Geometry: final body of the model. Coordinates: model frame, mm. A direction names the side the tool comes from. Round coordinates to 2 decimals unless told otherwise and drop trailing zeros. Loops run counter-clockwise (first coordinate to the right, second up) from the corner with the lowest first, then second, coordinate; pieces in that order, holes last. Notation, with made-up numbers: (36, 60) -> (78, 60) arc R5 cw to (78, 64) -> close; hole circle Ø1 at (19, 50). An arc over 180 degrees is marked (long way). Answer in a Markdown table with one row per item.
```python
from build123d import *

# Parameters (mm, degrees)
SKETCH1_W           = 30.1
SKETCH1_H           = 25.3
BOSS_EXTRUDE1_DEPTH = 1.1
SKETCH2_R           = 1.05
CUT_EXTRUDE1_DEPTH  = 2.1
SKETCH3_W           = 13
SKETCH3_H           = 13
BOSS_EXTRUDE2_DEPTH = 3
BOSS_EXTRUDE3_DEPTH = 3
SKETCH5_R           = 6.85
BOSS_EXTRUDE4_DEPTH = 20


with BuildPart() as part:
    # Sketch1 → Boss-Extrude1 (new body)
    with BuildSketch(Plane.XY):
        Rectangle(SKETCH1_W, SKETCH1_H)
    extrude(amount=BOSS_EXTRUDE1_DEPTH)

    # Sketch2 → Cut-Extrude1 (cut, through all)
    with BuildSketch(Plane.XY.offset(1.1)):
        with Locations((-11.8, 11.9)):
            Circle(SKETCH2_R)
        with Locations((11.8, 11.9)):
            Circle(SKETCH2_R)
        with Locations((11.8, -11.9)):
            Circle(SKETCH2_R)
        with Locations((-11.8, -11.9)):
            Circle(SKETCH2_R)
    extrude(amount=-CUT_EXTRUDE1_DEPTH, mode=Mode.SUBTRACT)

    # Sketch3 → Boss-Extrude2 (add)
    with BuildSketch(Plane.XY.offset(1.1)):
        Rectangle(SKETCH3_W, SKETCH3_H)
    extrude(amount=BOSS_EXTRUDE2_DEPTH)

    # Sketch4 → Boss-Extrude3 (add)
    with BuildSketch(Plane.XY.offset(1.1)):
        with BuildLine():
            Line((-8.9, 2), (8.9, 2))
            ThreePointArc((8.9, 2), (10.9, 0), (8.9, -2))
            Line((8.9, -2), (-8.9, -2))
            ThreePointArc((-8.9, -2), (-10.9, 0), (-8.9, 2))
        make_face()
    extrude(amount=BOSS_EXTRUDE3_DEPTH)

    # Sketch5 → Boss-Extrude4 (add)
    with BuildSketch(Plane.XY.offset(1.1)):
        Circle(SKETCH5_R)
    extrude(amount=BOSS_EXTRUDE4_DEPTH)


solid = part.part
```
Item 1: Pin query (flat end, axial travel): pin 1 Ø12 at (x, z) = (11.5, 12.5) entering from +Y; pin 2 Ø1.2 at (x, y) = (-9, 1) entering from +Z; pin 3 Ø3.5 at (x, y) = (-5, 5) entering from +Z; pin 4 Ø8 at (y, z) = (-2, 14) entering from -X. Return the tip coordinate at first contact, or that it passes through.
Answer:
| item | result |
|---|---|
| pin 1 | stops at y = 4.08 |
| pin 2 | stops at z = 4.1 |
| pin 3 | stops at z = 21.1 |
| pin 4 | stops at x = -6.85 |
Item 2: Cut plane C-C (y = 0). Output: boundary loops of the cut face in (x, z), then the cut area to 3 significant figures.
Answer:
| item | result |
|---|---|
| outline | (-15.05, 0) -> (15.05, 0) -> (15.05, 1.1) -> (10.9, 1.1) -> (10.9, 4.1) -> (6.85, 4.1) -> (6.85, 21.1) -> (-6.85, 21.1) -> (-6.85, 4.1) -> (-10.9, 4.1) -> (-10.9, 1.1) -> (-15.05, 1.1) -> close |
| area | 331 mm² |
Item 3: Cut plane D-D (x = 0). Output: boundary loops of the cut face in (y, z), then the cut area to 3 significant figures.
Answer:
| item | result |
|---|---|
| outline | (-12.65, 0) -> (12.65, 0) -> (12.65, 1.1) -> (6.85, 1.1) -> (6.85, 21.1) -> (-6.85, 21.1) -> (-6.85, 1.1) -> (-12.65, 1.1) -> close |
| area | 302 mm² |
Item 4: Line query: probe 1 along X at (y, z) = (11.9, 0.65); probe 2 along Y at (x, z) = (-2, 3.25); probe 3 along Z at (x, y) = (0, 8). Output: solid intervals per line, ascending. Write a range as [from, to].
Answer:
| item | result |
|---|---|
| probe 1 | x = [-15.05, -12.85], [-10.75, 10.75], [12.85, 15.05] |
| probe 2 | y = [-6.55, 6.55] |
| probe 3 | z = [0, 1.1] |
Item 5: Draft query along Y for faces 1 (the face through (-5, -5, 4.1)), 2 (the face through (13.8, -12.65, 0.5)), 3 (the face through (8, 2, 3)), 4 (the face through (11.83, -10.85, 0.56)). Return one class per face: pulls with the +Y half, pulls with the -Y half, needs draft (parallel to the pull), parting line crosses it, or undercut.
Answer:
| item | result |
|---|---|
| face 1 | needs draft |
| face 2 | pulls with the -Y half |
| face 3 | pulls with the +Y half |
| face 4 | undercut |
Item 6: Reachability of faces 5 (the face through (6.5, 4, 3)), 6 (the face through (-5, 5, 4.1)), 7 (the face through (5, -5, 4.1)), 8 (the face through (-0.2, -12.65, 0.5)), 9 (the face through (13.8, 12.65, 0.5)) from +Z, -Z, +X, -X, +Y, -Y: full face, straight path, thin tool, end or side. Return the list, or none.
Answer:
| item | result |
|---|---|
| face 5 | +Z, +X, +Y |
| face 6 | +Z, -X, +Y |
| face 7 | +Z, +X, -Y |
| face 8 | +Z, -Z, +X, -X, -Y |
| face 9 | +Z, -Z, +X, -X, +Y |
Item 7: Cut plane B-B (z = 3.25). Output: boundary loops of the cut face in (x, y).
Answer:
| item | result |
|---|---|
| outline | (-8.9, -2) -> (-6.55, -2) arc R6.85 ccw to (-6.5, -2.16) -> (-6.5, -6.5) -> (-2.16, -6.5) arc R6.85 ccw to (2.16, -6.5) -> (6.5, -6.5) -> (6.5, -2.16) arc R6.85 ccw to (6.55, -2) -> (8.9, -2) arc R2 ccw to (8.9, 2) -> (6.55, 2) arc R6.85 ccw to (6.5, 2.16) -> (6.5, 6.5) -> (2.16, 6.5) arc R6.85 ccw to (-2.16, 6.5) -> (-6.5, 6.5) -> (-6.5, 2.16) arc R6.85 ccw to (-6.55, 2) -> (-8.9, 2) arc R2 ccw to start |
Item 8: Cut plane A-A (y = 11.9). Output: boundary loops of the cut face in (x, z), then the cut area to 3 significant figures.
Answer:
| item | result |
|---|---|
| outline | (-15.05, 0) -> (-12.85, 0) -> (-12.85, 1.1) -> (-15.05, 1.1) -> close; (-10.75, 0) -> (10.75, 0) -> (10.75, 1.1) -> (-10.75, 1.1) -> close; (12.85, 0) -> (15.05, 0) -> (15.05, 1.1) -> (12.85, 1.1) -> close |
| area | 28.5 mm² |
